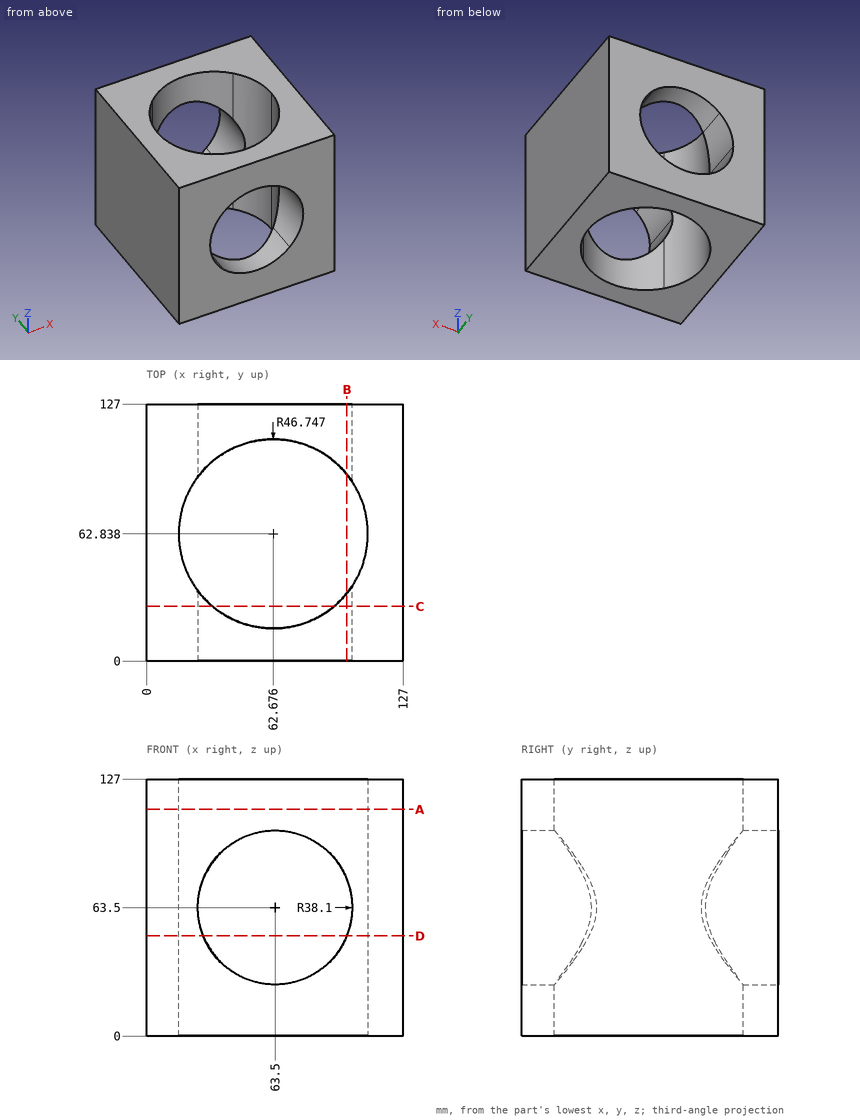
Verification items for this drawing (mm, ordinates from the low corner). Round coordinates to 2 decimals unless told otherwise and drop trailing zeros. Loops run counter-clockwise (first coordinate to the right, second up) from the corner with the lowest first, then second, coordinate; pieces in that order, holes last. Notation, with made-up numbers: (15, -25.5) -> (62, -25.5) arc R23 ccw to (62, -17.5) -> close; hole circle Ø9 at (-15.5, 75). An arc over 180 degrees is marked (long way). Write item = value, one per line. Start each with the question number.
1) Gauge pin test, flat end, axial feed: pin 1 Ø12 at (x, y) = (71, 100) entering from -Z. Record the tip position at first contact, or that the pin passes through.
2) Sectioned sample at C-C, the plane y = 27. Record the cut outline in (x, z) (1 decimal), plus the area to 3 significant figures.
3) Sectioned sample at D-D, the plane z = 49.5. Record the cut outline in (x, y) (1 decimal), plus the area to 3 significant figures.
4) Thickness scan on probe 1 along Y at (x, z) = (64.5, 102.5); probe 2 along Y at (x, z) = (24, 28) (1 decimal); probe 3 along X at (y, z) = (22, 98) (1 decimal). Record the ranges inside material, lowest first.
5) Sectioned sample at B-B, the plane x = 99. Record the cut outline in (y, z), plus the area to 3 significant figures.
6) Sectioned sample at A-A, the plane z = 112. Record the cut outline in (x, y) (1 decimal), plus the area to 3 significant figures.
Results are:
q1.pin_1 = through
q2.outline = (0, 0) -> (32.7, 0) -> (32.7, 41.1) arc R38.1 cw to (32.7, 85.9) -> (32.7, 127) -> (0, 127) -> close; (92.7, 0) -> (127, 0) -> (127, 127) -> (92.7, 127) -> (92.7, 88) arc R38.1 cw to (92.7, 39) -> close
q2.area = 7,990 mm^2
q3.outline = (0, 0) -> (28.1, 0) -> (28.1, 31.4) arc R46.7 cw to (28.1, 94.3) -> (28.1, 127) -> (0, 127) -> close; (98.9, 0) -> (127, 0) -> (127, 127) -> (98.9, 127) -> (98.9, 92.3) arc R46.7 cw to (109.4, 62.8) arc R46.7 cw to (98.9, 33.3) -> close
q3.area = 6,180 mm^2
q4.probe_1 = 0 to 16.13, 109.55 to 127
q4.probe_2 = 0 to 36.6, 89.1 to 127
q4.probe_3 = 0 to 39.9, 85.4 to 127
q5.outline = (0, 0) -> (33.41, 0) -> (33.41, 49.67) -> (0, 49.67) -> close; (0, 77.33) -> (33.41, 77.33) -> (33.41, 127) -> (0, 127) -> close; (92.26, 0) -> (127, 0) -> (127, 49.67) -> (92.26, 49.67) -> close; (92.26, 77.33) -> (127, 77.33) -> (127, 127) -> (92.26, 127) -> close
q5.area = 6,770 mm^2
q6.outline = (0, 0) -> (127, 0) -> (127, 127) -> (0, 127) -> close; hole (29.7, 29.7) arc R46.7 ccw to (95.6, 29.7) arc R46.7 ccw to (109.4, 62.8) arc R46.7 ccw to (95.7, 95.9) arc R46.7 ccw to start
q6.area = 9,260 mm^2
